Verification items for the finished model (mm, model axes). Round coordinates to 2 decimals unless told otherwise and drop trailing zeros. Order: outer loops, then holes, each group sorted by start corner. A loop starts at its lowest first (then second) coordinate and runs counter-clockwise, first axis right, second up. Notation, with made-up numbers: (33.25, 85.25) -> (88.25, 85.25) arc R14 cw to (88.25, 99.25) -> close; hole circle Ø3 at (78, -26.75). An arc over 180 degrees is marked (long way). Return JSON: item names as keys, results as strings. Group by question number.
Item 1: Sectioned sample at C-C on y = -38.5. Record the cut outline in (x, z).
Item 2: Depth check by flat-ended pin: pin 1 Ø5 at (x, y) = (13.87, 99.09) entering from +Z. Enter the tip coordinate at first touch or a pass-through.
Item 3: Draft check along X on faces 1 (the cylindrical face through (14.05, 102.265, 0.783)), 2 (the cylindrical face through (25.74, 120.24, 0.78)), 3 (the cylindrical face through (63.68, 46.07, 0.78)). Enter one of: pulls with the +X half, pulls with the -X half, needs draft (parallel to the pull), parting line crosses it, or undercut.
Item 4: Sectioned sample at D-D on x = 52.5. Record the cut outline in (y, z).
Item 5: Scan lines: probe 1 along Y at (x, z) = (14.5, 0.3); probe 2 along X at (y, z) = (-22.5, 0.7); probe 3 along Y at (x, z) = (-14, 0.15). Record each from-to range of solid material in increasing order. Write a range as from..to.
Item 6: Sectioned sample at A-A on x = 15. Record the cut outline in (y, z), plus the area to 3 significant figures.
Autodesk Inventor part; units mm, degrees
ref_plane "YZ Plane" through (0, 0, 0) normal (1, 0, 0) x (0, 1, 0)
ref_plane "XZ Plane" through (0, 0, 0) normal (0, 1, 0) x (-1, 0, 0)
ref_plane "XY Plane" through (0, 0, 0) normal (0, 0, 1) x (1, 0, 0)
ref_plane "Work Plane1" through (-99.6499, 20.9204, 0) normal (0, 0, 1) x (0.9625, -0.2713, 0)
sketch "Sketch1" plane through (-99.6499, 20.9204, 0) normal (0, 0, 1) x (0.9625, -0.2713, 0)
  arc A0 (85.2738, 81.502) -> (83.0074, 84.6783) centre (85.432, 84.0117) ccw construction
  circle A1 centre (88.0557, 106.0406) radius 3.175
  arc A2 (111.4983, 99.8389) -> (64.6131, 112.2422) centre (88.0557, 106.0406) ccw
  circle A3 centre (90.0577, 33.4227) radius 3.175 construction
  circle A4 centre (94.6835, -17.1663) radius 3.175 construction
  arc A5 (165.3065, -1.1832) -> (158.0816, 17.8159) centre (94.6835, -17.1663) ccw
  circle A6 centre (90.0577, 33.4227) radius 4.1833
  circle A7 centre (94.6835, -17.1663) radius 4.0324
  arc A8 (158.0816, 17.8159) -> (111.4983, 99.8389) centre (90.0577, 33.4227) ccw
  arc A9 (64.6131, 112.2422) -> (165.3065, -1.1832) centre (90.0577, 33.4227) ccw
  point P0 (101.5885, 6.8942)
  dimension "d0" = 6.35
extrude "Extrusion1" add sketch "Sketch1" along normal blind 1.5875
properties part number "driveGearSupportLayer"
Recorded:
{
 "1": {"outline": "(-52.38, 0) -> (44.57, 0) -> (44.57, 1.59) -> (-52.38, 1.59) -> close"},
 "2": {"pin 1": "through"},
 "3": {"face 1": "undercut", "face 2": "parting line crosses it", "face 3": "pulls with the +X half"},
 "4": {"outline": "(-32, 0) -> (69.76, 0) -> (69.76, 1.59) -> (-32, 1.59) -> close"},
 "5": {"probe 1": "-52.1..95.98, 102.21..123.34", "probe 2": "-69.04..-17.02, -9.33..59.22", "probe 3": "-53.55..-25.24, -17.34..110.86"},
 "6": {"outline": "(-51.98, 0) -> (96.13, 0) -> (96.13, 1.59) -> (-51.98, 1.59) -> close; (102.06, 0) -> (123.32, 0) -> (123.32, 1.59) -> (102.06, 1.59) -> close", "area": "269 mm²"}
}
